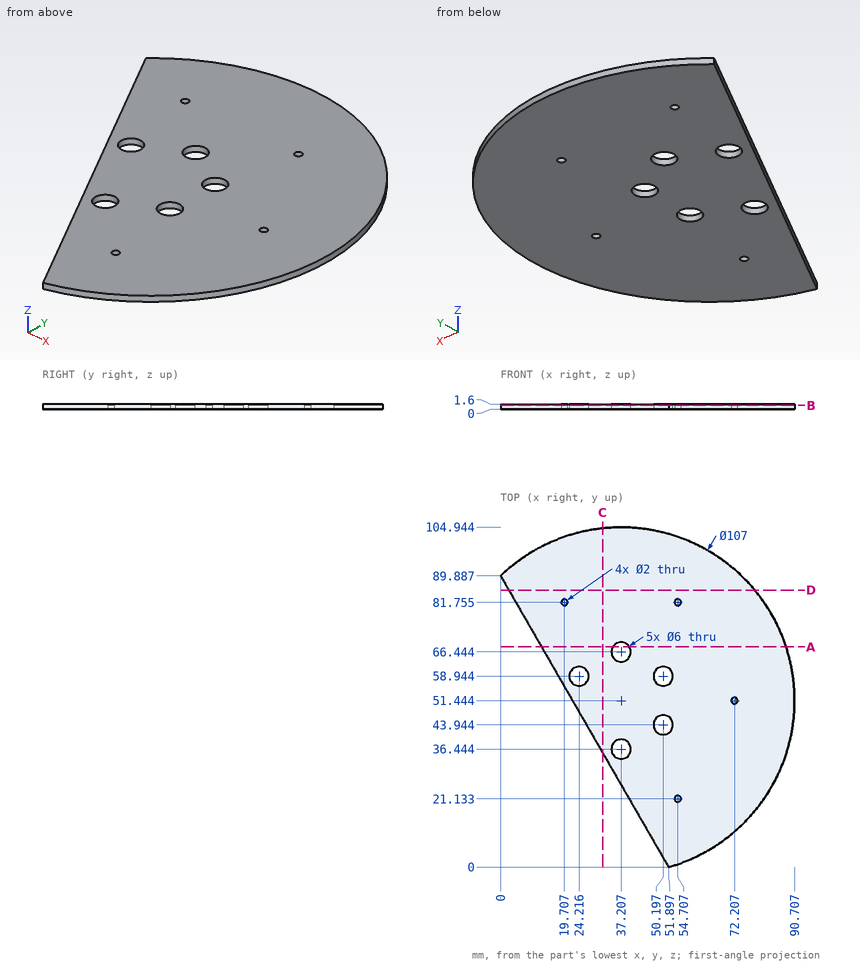
Input: dimensioned drawing with shaded views. Units: mm. Origin: part minimum x, y, z. Round coordinates to 2 decimals unless told otherwise and drop trailing zeros. Loops run counter-clockwise (first coordinate to the right, second up) from the corner with the lowest first, then second, coordinate; pieces in that order, holes last. Notation, with made-up numbers: M 5,61.5 L 34,61.5 A20 cw 34,95.5 Z; hole C 43,-22.5 d10. An arc over 180 degrees is marked long. Answer in a Markdown table with one row per item. Add a question column.
1. Section B-B (z = 1.2). Give the number of separate pieces and of enclosed holes in the cut face, and give its area (3 significant figures).
2. Contact query for a flat-ended pin moving along its axis: pin 1 (9.5 mm diameter, centred on x = 24.22, y = 58.94, fed in from +Z). Output: stop coordinate, or through.
3. Ray query, probe 1 along Y at (x, z) = (86, 1.4) (1 decimal); probe 2 along Y at (x, z) = (41, 0.9) (1 decimal); probe 3 along X at (y, z) = (13, 0.8) (1 decimal). Return the intervals inside material, ascending.
4. Section C-C (x = 31.5). Output: boundary loops of the cut face in (y, z), and give its area (3 significant figures).
5. Section A-A (y = 68). Output: boundary loops of the cut face in (x, z).
6. Section D-D (y = 85.5). Output: boundary loops of the cut face in (x, z).
Values follow:
| question | item | result |
|---|---|---|
| 1 | separate pieces | 1 |
| 1 | enclosed holes | 9 |
| 1 | area | 5,720 mm^2 |
| 2 | pin 1 | z = 1.6 |
| 3 | probe 1 | 29.5 to 73.4 |
| 3 | probe 2 | 18.9 to 104.8 |
| 3 | probe 3 | 44.4 to 74.4 |
| 4 | outline | M 35.33,0 L 104.64,0 L 104.64,1.6 L 35.33,1.6 Z |
| 4 | area | 111 mm^2 |
| 5 | outline | M 12.64,0 L 34.64,0 L 34.64,1.6 L 12.64,1.6 Z; M 39.77,0 L 88.08,0 L 88.08,1.6 L 39.77,1.6 Z |
| 6 | outline | M 2.53,0 L 78.47,0 L 78.47,1.6 L 2.53,1.6 Z |
